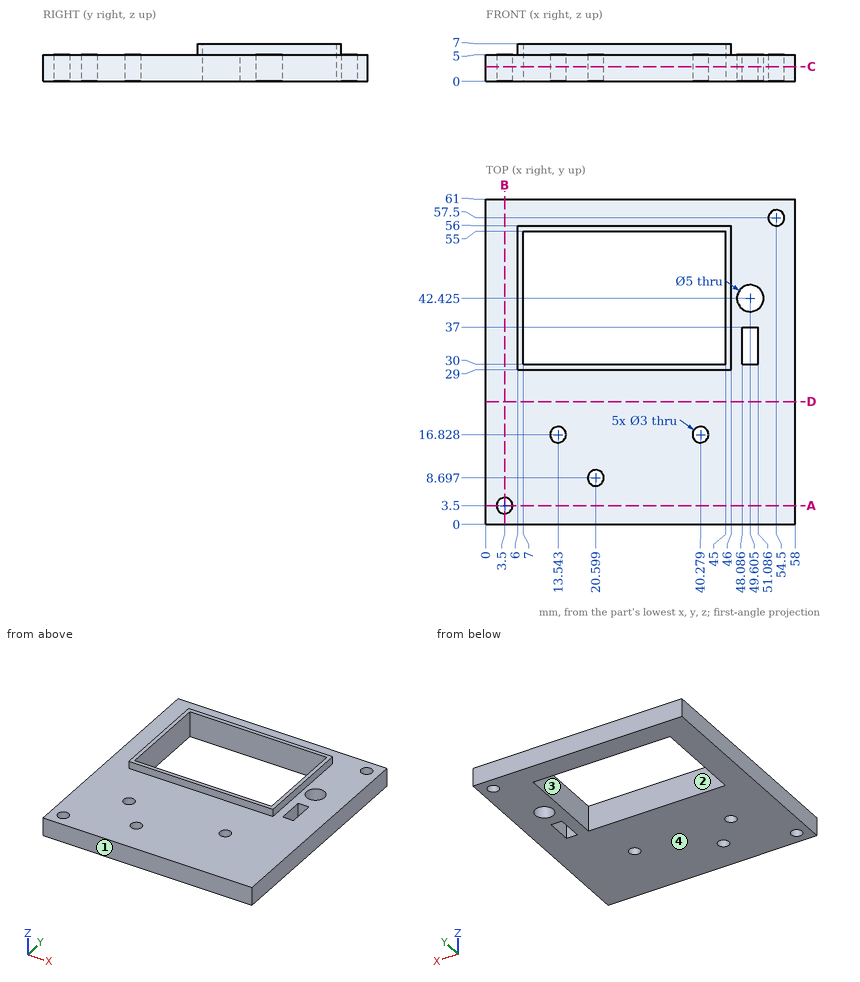
Geometry: see drawing. Coordinates: mm, zero at the bounding-box minimum. A direction names the side the tool comes from. Coordinates: 2 decimals unless noted, no trailing zeros. Write each loop counter-clockwise with the first axis right and the second up, starting at its lowest first coordinate (ties: lowest second). Pieces come first, ordered by that corner, then holes. Notation, with made-up numbers: M 24.5,3 L 68.5,3 A10 cw 68.5,15 Z; hole C 65,60 d8. An arc over 180 degrees is marked long. Answer as a JSON object with one key per item and string values.
1. Cut plane D-D on y = 23. Output: boundary loops of the cut face in (x, z).
Evaluation:
{"outline": "M 0,0 L 58,0 L 58,5 L 0,5 Z"}
2. Ray query, L1, parallel to X at y = 30.5, z = 0.5; L2, parallel to Y at x = 40.5, z = 2.5 (1 decimal); L3, parallel to X at y = 34, z = 6.5. Return the intervals inside material, ascending.
Evaluation:
{"L1": "0 to 7, 45 to 48.09, 51.09 to 58", "L2": "0 to 15.3, 18.3 to 30, 55 to 61", "L3": "6 to 7, 45 to 46"}
3. Contact query for flat-ended pins moving along their axis: P1, Ø1.6, axis at y = 42, z = 6, coming from the -X side; P2, Ø1, axis at x = 28.5, z = 6, coming from the +Y side; P3, Ø1.6, axis at y = 40, z = 6.5, coming from the +X side. Output: stop coordinate, or through.
Evaluation:
{"P1": "x = 6", "P2": "y = 56", "P3": "x = 46"}
4. Cut plane C-C on z = 2.75. State how many separate pieces and enclosed holes the cut face has, plus the area to 3 significant figures.
Evaluation:
{"separate pieces": "1", "enclosed holes": "8", "area": "2,510 mm^2"}
5. Cut plane A-A on y = 3.5. Output: boundary loops of the cut face in (x, z), plus the area to 3 significant figures.
Evaluation:
{"outline": "M 0,0 L 2,0 L 2,5 L 0,5 Z; M 5,0 L 58,0 L 58,5 L 5,5 Z", "area": "275 mm^2"}
6. Cut plane B-B on x = 3.5. Output: boundary loops of the cut face in (y, z), plus the area to 3 significant figures.
Evaluation:
{"outline": "M 0,0 L 2,0 L 2,5 L 0,5 Z; M 5,0 L 61,0 L 61,5 L 5,5 Z", "area": "290 mm^2"}
7. Draft query along X for the marked faces 3 and 4. Return one class per face: released by +X, released by -X, zero draft, split by the parting line, or undercut.
Evaluation:
{"face 3": "undercut", "face 4": "zero draft"}
8. Access query for the marked faces 1 and 2. Directions: +Z, -Z, +X, -X, +Y, -Y. A direction counts if a zero-diameter tool reaches every point of the face in a straight line with its end or side. Return the directions, or none.
Evaluation:
{"face 1": "+Z, -Z, +X, -X, -Y", "face 2": "+Z, -Z"}
